Build history of the part. All positions in model axes, mm. Face numbers are marked on the shaded views. A direction names the side the tool comes from. Give positions to 0.01 mm unless a question says otherwise; leave off trailing zeros. Write each loop counter-clockwise with the first axis right and the second up, starting at its lowest first coordinate (ties: lowest second). Pieces come first, ordered by that corner, then holes. Notation, with made-up numbers: M 16.25,-9 L 38.25,-9 A15 ccw 38.25,11 Z; hole C 16,16.5 d1. An arc over 180 degrees is marked long. Return JSON: item names as keys, results as strings. Group by question number.
Q1. Wall check: probe 1 along X at (y, z) = (30, 41) (3 decimals); probe 2 along Y at (x, z) = (14, 9.5). Give the ranges that are in metal, low to high.
Q2. Band-saw the part on A-A, the plane z = 53.5. Give the cut face in (x, y) (3 decimals), then the cut area to 3 significant figures.
Q3. Band-saw the part on D-D, the plane z = 38.1. Give the cut face in (x, y) (3 decimals), then the cut area to 3 significant figures.
Q4. Tool access for the marked faces 4 and 5: list every direction of +Z, -Z, +X, -X, +Y, -Y with a clear straight run to the whole face (end or side of a thin tool).
Q5. Pull direction Y, two halves, no side cores. Call the marked faces 1, 2 and 3: +Y half, -Y half, draft (parallel to the pull), parting line (faces both ways), or undercut.
Q6. Band-saw the part on B-B, the plane x = -31.5. Give the cut face in (y, z), then the cut area to 3 significant figures.
Q7. Band-saw the part on C-C, the plane y = -43.5. Give the cut face in (x, z) (3 decimals).
Q8. Flat gauge pins, fed straight in: pin 1 Ø3.5 at (x, y) = (-7.5, -61.5) entering from +Z; pin 2 Ø23 at (y, z) = (-6.82, 38.1) entering from +X. Where does each tip first touch, or does it go through?
from build123d import *

# Parameters (mm, degrees)
F0_W     = 139.7
F0_H     = 114.3
F0_W_2   = 133.35
F0_H_2   = 107.95
F1_DEPTH = 76.2
F2_W     = 50.8
F2_H     = 50.8
F3_DEPTH = 127
F4_R     = 12.7
F5_DEPTH = 175.768


with BuildPart() as f1:
    # F0 (on Top) → F1 (new body)
    with BuildSketch(Plane.XY):
        with Locations((0, -6.816931)):
            Rectangle(F0_W, F0_H)
        with Locations((0, -6.816931)):
            Rectangle(F0_W_2, F0_H_2, mode=Mode.SUBTRACT)
    extrude(amount=F1_DEPTH)

    # F2 (on face) → F3 (cut)
    with BuildSketch(Plane.XZ.offset(63.966931)):
        with Locations((0, 76.2)):
            Rectangle(F2_W, F2_H)
    extrude(amount=-F3_DEPTH, mode=Mode.SUBTRACT)

    # F4 (on face) → F5 (cut)
    with BuildSketch(Plane.YZ.offset(69.85)):
        with Locations((-6.816931, 38.1)):
            Circle(F4_R)
    extrude(amount=-F5_DEPTH, mode=Mode.SUBTRACT)


solid = f1.part
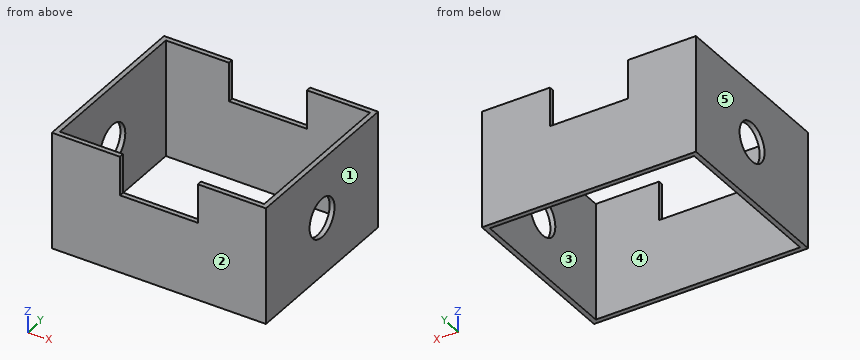
From the geometry:
{
 "1": {"probe 1": "x = -69.85 to -66.675, 66.675 to 69.85", "probe 2": "y = -63.97 to -60.79, 47.16 to 50.33"},
 "2": {"outline": "M -69.85,-63.967 L -25.4,-63.967 L -25.4,-60.792 L -66.675,-60.792 L -66.675,47.158 L -25.4,47.158 L -25.4,50.333 L -69.85,50.333 Z; M 25.4,-63.967 L 69.85,-63.967 L 69.85,50.333 L 25.4,50.333 L 25.4,47.158 L 66.675,47.158 L 66.675,-60.792 L 25.4,-60.792 Z", "area": "1,250 mm^2"},
 "3": {"outline": "M -69.85,-63.967 L 69.85,-63.967 L 69.85,-19.517 L 66.675,-19.517 L 66.675,-60.792 L -66.675,-60.792 L -66.675,-19.517 L -69.85,-19.517 Z; M -69.85,5.883 L -66.675,5.883 L -66.675,47.158 L 66.675,47.158 L 66.675,5.883 L 69.85,5.883 L 69.85,50.333 L -69.85,50.333 Z", "area": "1,410 mm^2"},
 "4": {"face 4": "+Z, -Z", "face 5": "+Z, -Z, -X, +Y, -Y"},
 "5": {"face 1": "draft", "face 2": "-Y half", "face 3": "undercut"},
 "6": {"outline": "M -63.97,0 L -60.79,0 L -60.79,76.2 L -63.97,76.2 Z; M 47.16,0 L 50.33,0 L 50.33,76.2 L 47.16,76.2 Z", "area": "484 mm^2"},
 "7": {"outline": "M -69.85,0 L -66.675,0 L -66.675,76.2 L -69.85,76.2 Z; M 66.675,0 L 69.85,0 L 69.85,76.2 L 66.675,76.2 Z"},
 "8": {"pin 1": "stops at z = 50.8", "pin 2": "passes through"}
}
